```python
from build123d import *

# Parameters (mm, degrees)
SKETCH1_R           = 6
SKETCH1_R_2         = 3.25
SKETCH1_R_3         = 4.25
BOSS_EXTRUDE2_DEPTH = 4.7625
FILLET1_R           = 9.53


with BuildPart() as part:
    # Sketch1 → Boss-Extrude2 (new body)
    with BuildSketch(Plane.XY):
        Polygon((-45.444705817, 407.184725354), (-95.444705817, 395.759725354), (-95.444705817, 376.709725354), (-45.444705817, 367.184725354), (34.555294183, 367.184725354), (80.755294183, 376.714725354), (80.755294183, 397.654725354), (30.755294183, 407.184725354), align=None)
        with Locations(Location((-29.244705817, 387.184725354, 0), (0, 0, 180))):
            Circle(SKETCH1_R, mode=Mode.SUBTRACT)
        with Locations(Location((10.755294183, 387.184725354, 0), (0, 0, 180))):
            Circle(SKETCH1_R_2, mode=Mode.SUBTRACT)
        with Locations(Location((-85.444705817, 386.234725354, 0), (0, 0, 180))):
            Circle(SKETCH1_R_3, mode=Mode.SUBTRACT)
        with Locations(Location((70.755294183, 388.134725354, 0), (0, 0, 180))):
            Circle(SKETCH1_R_3, mode=Mode.SUBTRACT)
    extrude(amount=BOSS_EXTRUDE2_DEPTH)

    # Fillet1
    fillet1_edges = [part.edges().sort_by_distance(p)[0] for p in [
        (-95.444705817, 376.709725354, 2.38125),
        (-95.444705817, 395.759725354, 2.38125),
        (-45.444705817, 407.184725354, 2.38125),
        (30.755294183, 407.184725354, 2.38125),
        (80.755294183, 397.654725354, 2.38125),
        (80.755294183, 376.714725354, 2.38125),
        (34.555294183, 367.184725354, 2.38125),
        (-45.444705817, 367.184725354, 2.38125),
    ]]
    fillet(fillet1_edges, radius=FILLET1_R)


solid = part.part
```
The model under review builds one solid part; all positions refer to its coordinate system, in mm. Round coordinates to 2 decimals unless told otherwise and drop trailing zeros. Order: outer loops, then holes, each group sorted by start corner. A loop starts at its lowest first (then second) coordinate and runs counter-clockwise, first axis right, second up. Notation, with made-up numbers: (49.25, 73.5) -> (103.25, 73.5) arc R19 cw to (103.25, 87.5) -> close; hole circle Ø5 at (15.5, 38). An arc over 180 degrees is marked (long way). One line per item, written item: value. Start each with the question number.
Q1. Clearance check with a flat-ended pin moving along its axis: pin 1 Ø1.5 at (x, z) = (52.5, 2) entering from -Y. State where the tip first meets the part, or that it passes through.
Q2. Mouldability with a two-part tool opening along Y and no side actions: class faces 1 (the face through (-82.312, 383.362, 2.348)), 2 (the face through (78.67, 378.53, 2.41)), 3 (the face through (-93.31, 394.17, 2.41)), 4 (the face through (-28.464, 381.236, 2.348)) as released by +Y, released by -Y, zero draft, split by the parting line, or undercut.
Q3. Take a section at B-B (z = 3.1). Write out the cut boundary in (x, y), and give its area (3 significant figures).
Q4. Wall thickness on line 1 (X direction, y = 386.5, z = 1.35); line 2 (X direction, y = 392, z = 2.6); line 3 (Y direction, x = 10.5, z = 4.3): over which ranges is each line inside the solid? List them lowest first.
Q5. Take a section at C-C (y = 395.5). Write out the cut boundary in (x, z).
Q6. Take a section at A-A (x = -28.5). Write out the cut boundary in (y, z), and give its area (3 significant figures).
Reported:
1. pin 1: stops at y = 370.73
2. face 1: undercut
2. face 2: released by -Y
2. face 3: released by +Y
2. face 4: undercut
3. outline: (-95.44, 384.6) arc R9.53 ccw to (-87.7, 375.23) -> (-46.33, 367.35) arc R9.53 ccw to (-44.55, 367.18) -> (33.58, 367.18) arc R9.53 ccw to (35.51, 367.38) -> (73.15, 375.15) arc R9.53 ccw to (80.76, 384.48) -> (80.76, 389.77) arc R9.53 ccw to (73.01, 399.13) -> (31.64, 407.02) arc R9.53 ccw to (29.86, 407.18) -> (-44.37, 407.18) arc R9.53 ccw to (-46.49, 406.95) -> (-88.04, 397.45) arc R9.53 ccw to (-95.44, 388.16) -> close; hole circle Ø8.5 at (-85.44, 386.23); hole circle Ø12 at (-29.24, 387.18); hole circle Ø6.5 at (10.76, 387.18); hole circle Ø8.5 at (70.76, 388.13)
3. area: 5,760 mm2
4. line 1: x = -95.44 to -89.69, -81.2 to -35.21, -23.28 to 7.58, 13.93 to 66.83, 74.68 to 80.76
4. line 2: x = -94.64 to -32.82, -25.67 to 68.99, 72.52 to 80.49
4. line 3: y = 367.18 to 383.94, 390.42 to 407.18
5. outline: (-92, 0) -> (78.84, 0) -> (78.84, 4.76) -> (-92, 4.76) -> close
6. outline: (367.18, 0) -> (381.23, 0) -> (381.23, 4.76) -> (367.18, 4.76) -> close; (393.14, 0) -> (407.18, 0) -> (407.18, 4.76) -> (393.14, 4.76) -> close
6. area: 134 mm2
